```python
from build123d import *

# Parameters (mm, degrees)
F0_W     = 25
F0_H     = 50
F1_DEPTH = 75
F2_DEPTH = 50
F3_DEPTH = 75


with BuildPart() as f1:
    # F0 (on Top) → F1 (new body)
    with BuildSketch(Plane.XY):
        with Locations((12.5, 25)):
            Rectangle(F0_W, F0_H)
    extrude(amount=F1_DEPTH)

    # F0 (on Top) → F2 (join)
    with BuildSketch(Plane.XY):
        Polygon((25, 50), (25, 0), (42.5, 0), (42.5, 15), (65, 15), (65, 10), (85, 10), (85, 50), align=None)
    extrude(amount=F2_DEPTH)

    # F0 (on Top) → F3 (join)
    with BuildSketch(Plane.XY):
        Polygon((115, 50), (85, 50), (85, 10), (95, 10), (95, -20), (115, -20), align=None)
    extrude(amount=F3_DEPTH)


solid = f1.part
```
Check sheet for the modelled part. Datum: model origin and axes. Units: mm. A direction names the side the tool comes from. Give positions to 0.01 mm unless a question says otherwise; leave off trailing zeros. Order: outer loops, then holes, each group sorted by start corner. A loop starts at its lowest first (then second) coordinate and runs counter-clockwise, first axis right, second up. Notation, with made-up numbers: M 66,14.5 L 96,14.5 A32 ccw 96,46.5 Z; hole C -6,25.25 d7. An arc over 180 degrees is marked long. Answer in a Markdown table with one row per item. Add a question column.
Q1. Access from +Z, -Z, +X, -X, +Y, -Y to the whole of each face (thin tool, end or side, straight path). Record for faces 5 (the flat face through (55, 31, 50)), 6 (the flat face through (21, 0, 29)), 7 (the flat face through (80, 10, 29)).
Q2. Sectioned sample at B-B, the plane z = 66. Record the boundary of the cut face in (x, y).
Q3. Release check for a two-part mould opening along X. For faces 1 (the flat face through (95, -5, 37)), 2 (the flat face through (25, 25, 62)), 3 (the flat face through (0, 25, 37)), 4 (the flat face through (115, 15, 37)) record: released by +X, released by -X, zero draft, split by the parting line, or undercut.
Q4. Gauge pin test, flat ends, axial feed: pin 1 Ø9 at (y, z) = (-7.5, 47) entering from -X; pin 2 Ø1.5 at (x, y) = (36.5, 41.5) entering from +Z; pin 3 Ø18 at (x, z) = (50.5, 28) entering from -Y; pin 4 Ø2.5 at (y, z) = (12, 14.5) entering from -X. Record the tip position at first contact, or that the pin passes through.
Q5. Sectioned sample at A-A, the plane y = 5.5. Record the boundary of the cut face in (x, z).
Q6. Sectioned sample at D-D, the plane y = 41. Record the boundary of the cut face in (x, z).
Q7. Sectioned sample at C-C, the plane z = 22. Record the boundary of the cut face in (x, y), and give its area (3 significant figures).
Q8. Thickness scan on L1, parallel to X at y = 46.5, z = 60.5; L2, parallel to X at y = 14, z = 44; L3, parallel to Z at x = 35, y = 18.5. Record the ranges inside material, lowest first.
Verdict:
| question | item | result |
|---|---|---|
| 1 | face 5 | +Z, +Y, -Y |
| 1 | face 6 | +Z, -Z, -X, -Y |
| 1 | face 7 | +Z, -Z, -Y |
| 2 | outline | M 0,0 L 25,0 L 25,50 L 0,50 Z; M 85,10 L 95,10 L 95,-20 L 115,-20 L 115,50 L 85,50 Z |
| 3 | face 1 | undercut |
| 3 | face 2 | undercut |
| 3 | face 3 | released by -X |
| 3 | face 4 | released by +X |
| 4 | pin 1 | x = 95 |
| 4 | pin 2 | z = 50 |
| 4 | pin 3 | y = 0 |
| 4 | pin 4 | x = 0 |
| 5 | outline | M 0,0 L 42.5,0 L 42.5,50 L 25,50 L 25,75 L 0,75 Z; M 95,0 L 115,0 L 115,75 L 95,75 Z |
| 6 | outline | M 0,0 L 115,0 L 115,75 L 85,75 L 85,50 L 25,50 L 25,75 L 0,75 Z |
| 7 | outline | M 0,0 L 42.5,0 L 42.5,15 L 65,15 L 65,10 L 95,10 L 95,-20 L 115,-20 L 115,50 L 0,50 Z |
| 7 | area | 5,510 mm² |
| 8 | L1 | 0 to 25, 85 to 115 |
| 8 | L2 | 0 to 42.5, 65 to 115 |
| 8 | L3 | 0 to 50 |
